Verification items for the finished model (mm, model axes). Face numbers are marked on the shaded views. Give positions to 0.01 mm unless a question says otherwise; leave off trailing zeros. Loops run counter-clockwise (first coordinate to the right, second up) from the corner with the lowest first, then second, coordinate; pieces in that order, holes last. Notation, with made-up numbers: M 58,44 L 109,44 A31 cw 109,74 Z; hole C -9.75,-19 d3. An arc over 180 degrees is marked long. Answer in a Markdown table with one row per item.
```python
from build123d import *

# Parameters (mm, degrees)
F0_W     = 87.075323
F0_H     = 90.703461
F1_DEPTH = 63.246
F2_R     = 10.983628
F3_DEPTH = 25.4
F4_R     = 17.151938
F5_DEPTH = 25.4


with BuildPart() as f1:
    # F0 (on Top) → F1 (new body)
    with BuildSketch(Plane.XY):
        with Locations((6.969846, -0.381911)):
            Rectangle(F0_W, F0_H)
    extrude(amount=F1_DEPTH)

    # F2 (on Top) → F3 (cut)
    with BuildSketch(Plane.XY):
        Circle(F2_R)
    extrude(amount=-F3_DEPTH, mode=Mode.SUBTRACT)

    # F4 (on face) → F5 (cut)
    with BuildSketch(Plane.XZ.offset(45.733642)):
        with Locations((2.386932, 35.803996)):
            Circle(F4_R)
    extrude(amount=-F5_DEPTH, mode=Mode.SUBTRACT)


solid = f1.part
```
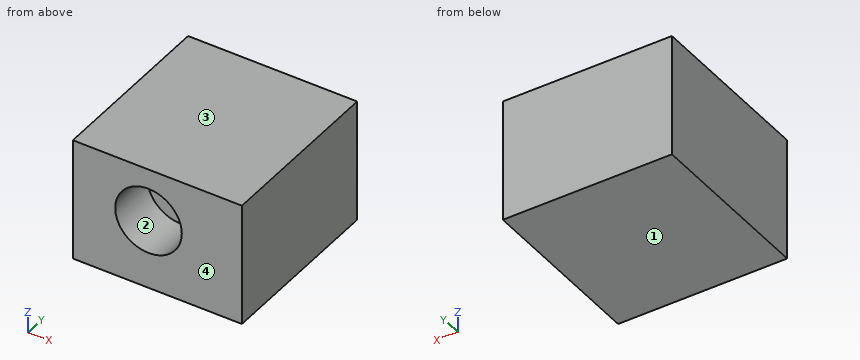
Item 1: Sectioned sample at B-B (x = 16). Record the cut outline in (y, z).
Reported:
| item | result |
|---|---|
| outline | M -45.73,0 L 44.97,0 L 44.97,63.25 L -45.73,63.25 L -45.73,46.24 L -20.33,46.24 L -20.33,25.37 L -45.73,25.37 Z |
Item 2: Sectioned sample at C-C (y = -28). Record the cut outline in (x, z), and give its area (3 significant figures).
Reported:
| item | result |
|---|---|
| outline | M -36.57,0 L 50.51,0 L 50.51,63.25 L -36.57,63.25 Z; hole C 2.39,35.8 d34.3 |
| area | 4,580 mm^2 |
Item 3: Go/stop test with a flat-tipped pin: pin 1 (8 mm diameter, centred on x = 7, z = 43, fed in from -Y). Record where the tip stops, or that it passes through.
Reported:
| item | result |
|---|---|
| pin 1 | stops at y = -20.33 |
Item 4: Scan lines: L1, parallel to Y at x = 12, z = 40; L2, parallel to X at y = -28, z = 45; L3, parallel to Z at x = 4.5, y = -23. Record each from-to range of solid material in increasing order. Write a range as [from, to].
Reported:
| item | result |
|---|---|
| L1 | y = [-20.33, 44.97] |
| L2 | x = [-36.57, -12.09], [16.87, 50.51] |
| L3 | z = [0, 18.78], [52.83, 63.25] |
Item 5: Release check for a two-part mould opening along Z. For the marked faces 1, 2, 3 and 4 record: released by +Z, released by -Z, zero draft, split by the parting line, or undercut.
Reported:
| item | result |
|---|---|
| face 1 | released by -Z |
| face 2 | undercut |
| face 3 | released by +Z |
| face 4 | zero draft |
Item 6: Sectioned sample at A-A (z = 40.5). Record the cut outline in (x, y).
Reported:
| item | result |
|---|---|
| outline | M -36.57,-45.73 L -14.11,-45.73 L -14.11,-20.33 L 18.88,-20.33 L 18.88,-45.73 L 50.51,-45.73 L 50.51,44.97 L -36.57,44.97 Z |
